Design review of the part shown in the three views and the two pictorial views. Dimensions are in mm from the part's minimum x, y and z. Round coordinates to 2 decimals unless told otherwise and drop trailing zeros. Loops run counter-clockwise (first coordinate to the right, second up) from the corner with the lowest first, then second, coordinate; pieces in that order, holes last. Notation, with made-up numbers: (89, 27.5) -> (107, 27.5) arc R33 cw to (107, 61.5) -> close; hole circle Ø8 at (67, 34.5). An arc over 180 degrees is marked (long way). Write each question's results on one line, items separated by ' | '. Start each with the question number.
Item 1: We need section B-B (x = 50). Give the boundary of the cut face in (y, z).
Item 2: Clearance check with flat-ended pins moving along their axes: pin 1 Ø5 at (x, y) = (54.5, 2.5) entering from +Z; pin 2 Ø2.5 at (x, z) = (17.12, 82.88) entering from -Y; pin 3 Ø1.5 at (y, z) = (3, 35.5) entering from +X. State where each tip first meets the part, or that it passes through.
Item 3: For L1, parallel to Z at x = 50, y = 0.5; L2, parallel to X at y = 7.5, z = 84 (1 decimal); L3, parallel to X at y = 5.25, z = 54.5 (1 decimal), list the stretches that pass through material, from the lowest coordinate up. Write a range as from..to.
Item 4: We need section C-C (y = 2.25). Give the boundary of the cut face in (x, z).
Item 5: Mouldability with a two-part tool opening along X and no side actions: class the marked faces 1, 2 and 3 as pulls with the +X half, pulls with the -X half, needs draft (parallel to the pull), parting line crosses it, or undercut.
Item 6: We need section A-A (z = 50). Give the boundary of the cut face in (x, y).
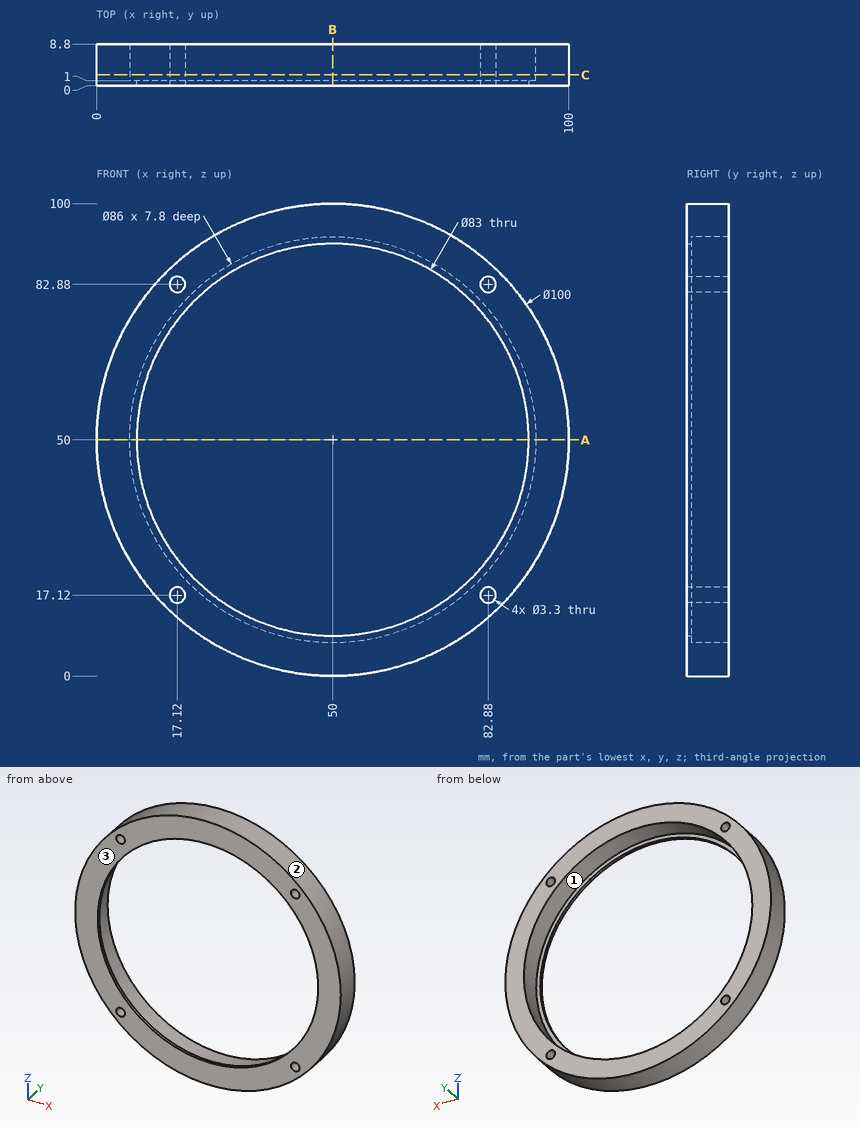
Here are the results:
1) outline: (0, 0) -> (8.8, 0) -> (8.8, 7) -> (1, 7) -> (1, 8.5) -> (0, 8.5) -> close; (0, 91.5) -> (1, 91.5) -> (1, 93) -> (8.8, 93) -> (8.8, 100) -> (0, 100) -> close
2) pin 1: stops at z = 99.96 | pin 2: passes through | pin 3: stops at x = 98.07
3) L1: z = 0..8.5, 91.5..100 | L2: x = 13.3..15.9, 18.3..23.7, 76.3..81.7, 84.1..86.7 | L3: x = 0.2..7.2, 92.8..99.8
4) outline: circle Ø100 at (50, 50); hole circle Ø86 at (50, 50); hole circle Ø3.3 at (17.12, 17.12); hole circle Ø3.3 at (17.12, 82.88); hole circle Ø3.3 at (82.88, 17.12); hole circle Ø3.3 at (82.88, 82.88)
5) face 1: undercut | face 2: parting line crosses it | face 3: needs draft
6) outline: (0, 0) -> (8.5, 0) -> (8.5, 1) -> (7, 1) -> (7, 8.8) -> (0, 8.8) -> close; (91.5, 0) -> (100, 0) -> (100, 8.8) -> (93, 8.8) -> (93, 1) -> (91.5, 1) -> close
